Input: part model. Units: mm. Frame: model coordinates. Face numbers are marked on the shaded views. A direction names the side the tool comes from. Give positions to 0.01 mm unless a question says otherwise; leave off trailing zeros. Order: outer loops, then holes, each group sorted by start corner. A loop starts at its lowest first (then second) coordinate and runs counter-clockwise, first axis right, second up. Notation, with made-up numbers: (13.5, -29) - (50.5, -29) arc R22 cw to (50.5, -21) - close; hole circle Ø11 at (2, -3). An arc over 180 degrees is marked (long way). Answer in a Markdown table with one row per item. Add a question column.
from build123d import *

# Parameters (mm, degrees)
SKETCH1_R           = 17.5
BOSS_EXTRUDE1_DEPTH = 63
CUT_EXTRUDE1_START  = -35
CUT_EXTRUDE1_DEPTH  = 35


with BuildPart() as part:
    # Sketch1 → Boss-Extrude1 (new body)
    with BuildSketch(Plane(origin=(0, 0, 0), x_dir=(1, 0, 0), z_dir=(0, 1, 0))):
        with Locations(Location((0, 0, 0), (0, 0, 270))):
            Circle(SKETCH1_R)
    extrude(amount=BOSS_EXTRUDE1_DEPTH)

    # Sketch2 → Cut-Extrude1 (cut)
    with BuildSketch(Plane(origin=(0, 63, 0), x_dir=(1, 0, 0), z_dir=(0, 1, 0)).offset(CUT_EXTRUDE1_START)):
        with BuildLine():
            Line((-5, 12.5), (5, 12.5))
            Line((5, 12.5), (5, 16.770509831))
            ThreePointArc((5, 16.770509831), (0, 17.5), (-5, 16.770509831))
            Line((-5, 16.770509831), (-5, 12.5))
        make_face()
    extrude(amount=CUT_EXTRUDE1_DEPTH, mode=Mode.SUBTRACT)


solid = part.part
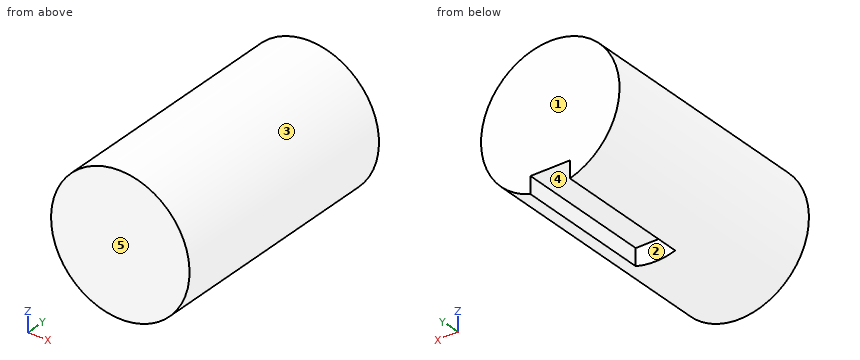
Q1. Access query for the marked faces 1 and 2. Directions: +Z, -Z, +X, -X, +Y, -Y. A direction counts if a zero-diameter tool reaches every point of the face in a straight line with its end or side. Return the directions, or none.
Q2. Contact query for flat-ended pins moving along their axis: P1, Ø2, axis at y = 47.5, z = -14, coming from the +X side; P2, Ø11, axis at x = -2, y = 40, coming from the -Z side; P3, Ø6, axis at y = 30, z = -7.5, coming from the -X side; P4, Ø4, axis at y = 33.5, z = -1, coming from the +X side. Output: stop coordinate, or through.
Q3. Pull-direction query (X, two-part tool) for the marked faces 3, 4 and 5; classes: +X half, -X half, draft (parallel to the pull), parting line (faces both ways), or undercut.
Q4. Section C-C, the plane y = 42. Return loops of the section in (x, z).
Q5. Section A-A, the plane z = -14. Return loops of the section in (x, y), then the cut area to 3 significant figures.
Q6. Line query: probe 1 along X at (y, z) = (17, 0.5); probe 2 along Z at (x, y) = (-16, 17); probe 3 along X at (y, z) = (37, 4). Output: solid intervals per line, ascending.
Q7. Section D-D, the plane x = 4. Return loops of the section in (y, z).
Q8. Section B-B, the plane x = 0. Return loops of the section in (y, z), then the cut area to 3 significant figures.
Computed:
| question | item | result |
|---|---|---|
| 1 | face 1 | +Z, -Z, +X, -X, +Y |
| 1 | face 2 | -Z, +Y |
| 2 | P1 | stops at x = 11.72 |
| 2 | P2 | stops at z = -16.77 |
| 2 | P3 | stops at x = -16.91 |
| 2 | P4 | stops at x = 17.5 |
| 3 | face 3 | parting line |
| 3 | face 4 | undercut |
| 3 | face 5 | draft |
| 4 | outline | (-5, -16.77) - (-5, -12.5) - (5, -12.5) - (5, -16.77) arc R17.5 ccw (long way) to start |
| 5 | outline | (-10.5, 0) - (10.5, 0) - (10.5, 63) - (5, 63) - (5, 28) - (-5, 28) - (-5, 63) - (-10.5, 63) - close |
| 5 | area | 973 mm^2 |
| 6 | probe 1 | x = -17.49 to 17.49 |
| 6 | probe 2 | z = -7.09 to 7.09 |
| 6 | probe 3 | x = -17.04 to 17.04 |
| 7 | outline | (0, -17.04) - (28, -17.04) - (28, -12.5) - (63, -12.5) - (63, 17.04) - (0, 17.04) - close |
| 8 | outline | (0, -17.5) - (28, -17.5) - (28, -12.5) - (63, -12.5) - (63, 17.5) - (0, 17.5) - close |
| 8 | area | 2,030 mm^2 |
